from build123d import *

# Parameters (mm, degrees)
EXTRUDE_1_DEPTH = 25
SKETCH_2_W      = 22.6
SKETCH_2_H      = 10
EXTRUDE_2_DEPTH = 15
FILLET_1_R      = 1


with BuildPart() as part:
    # 草图1 → 凸台-拉伸1 (new body)
    with BuildSketch(Plane(origin=(0, 0, 0), x_dir=(1, 0, 0), z_dir=(0, 1, 0))):
        with BuildLine():
            Line((0, 0), (22.6, 0))
            ThreePointArc((22.6, 0), (25.428427125, 1.171572875), (26.6, 4))
            Line((26.6, 4), (26.6, 84))
            Line((26.6, 84), (34.6, 84))
            Line((34.6, 84), (34.6, 4))
            ThreePointArc((34.6, 4), (31.085281374, -4.485281374), (22.6, -8))
            Line((22.6, -8), (0, -8))
            Line((0, -8), (0, 0))
        make_face()
    extrude(amount=EXTRUDE_1_DEPTH)

    # 草图2 → 凸台-拉伸2 (add)
    with BuildSketch(Plane.XY.offset(8)):
        with Locations((11.3, 20)):
            Rectangle(SKETCH_2_W, SKETCH_2_H)
    extrude(amount=EXTRUDE_2_DEPTH)

    # 圆角1
    fillet_1_edges = [part.edges().sort_by_distance(p)[0] for p in [
        (0, 25, 11.5),
        (0, 12.5, 0),
        (0, 7.5, 8),
        (0, 15, 15.5),
        (0, 20, 23),
    ]]
    fillet(fillet_1_edges, radius=FILLET_1_R)


solid = part.part
Can you work these out from the model? Positions are in its coordinate system, mm. A direction names the side the tool comes from. Give positions to 0.01 mm unless a question says otherwise; leave off trailing zeros. Order: outer loops, then holes, each group sorted by start corner. A loop starts at its lowest first (then second) coordinate and runs counter-clockwise, first axis right, second up. Notation, with made-up numbers: M 26,87 L 59,87 A16 cw 59,95 Z; hole C 18,-19 d6. An arc over 180 degrees is marked long. Use one line per item in the form item = value. Start each with the question number.
Item 1: For faces 1 (the flat face through (29, 25, -19)), 2 (the flat face through (26.6, 12, -43)), 3 (the flat face through (22.6, 20, 15)), 4 (the flat face through (28, 0, -31)), 5 (the flat face through (12, 7, 8)), which set-ups out of +Z, -Z, +X, -X, +Y, -Y let a thin tool reach every point of the face, with its end or its side?
Item 2: If we section it at A-A (y = 13.75): Write out the boundary of the cut face in (x, z), then the cut area to 3 significant figures.
Item 3: If we section it at C-C (z = 6): Write out the boundary of the cut face in (x, y), then the cut area to 3 significant figures.
Item 4: If I drill on line 1 along Z through (x, y) = (6, 17.75); line 2 along Y through (x, z) = (22.5, 14.5); line 3 along Z through (x, y) = (14.5, 3), over which ranges is the centre line in solid material (lowest first)?
Item 5: If we section it at D-D (z = -21): Write out the boundary of the cut face in (x, y).
Item 6: Will these pins go through, and if not, where does the flat tip stop? pin 1 Ø6 at (x, y) = (26, 21) entering from +Z; pin 2 Ø3 at (y, z) = (19.5, 18) entering from +X; pin 3 Ø6.5 at (x, y) = (8, 16.5) entering from -Z.
Item 7: If we section it at B-B (x = 17): Write out the boundary of the cut face in (y, z).
Outcome:
q1.face_1 = +Z, -Z, +X, -X, +Y
q1.face_2 = -Z, -X, +Y, -Y
q1.face_3 = +Z, +X, +Y, -Y
q1.face_4 = +Z, -Z, +X, -X, -Y
q1.face_5 = +Z, +X, -X, -Y
q2.outline = M 0,1 A1 ccw 1,0 L 22.6,0 A4 cw 26.6,-4 L 26.6,-84 L 34.6,-84 L 34.6,-4 A12 ccw 22.6,8 L 1,8 A1 ccw 0,7 Z
q2.area = 921 mm2
q3.outline = M 0,0 L 29.23,0 L 29.23,25 L 1,25 A1 ccw 0,24 Z
q3.area = 731 mm2
q4.line_1 = 0 to 23
q4.line_2 = 15 to 25
q4.line_3 = 0 to 8
q5.outline = M 26.6,0 L 34.6,0 L 34.6,25 L 26.6,25 Z
q6.pin_1 = 7.99
q6.pin_2 = 22.6
q6.pin_3 = 0
q7.outline = M 0,0 L 25,0 L 25,23 L 15,23 L 15,8 L 0,8 Z
